Check sheet for the modelled part. Datum: model origin and axes. Units: mm. A direction names the side the tool comes from. Round coordinates to 2 decimals unless told otherwise and drop trailing zeros. Order: outer loops, then holes, each group sorted by start corner. A loop starts at its lowest first (then second) coordinate and runs counter-clockwise, first axis right, second up. Notation, with made-up numbers: (-12, 85.25) -> (35, 85.25) arc R33 ccw to (35, 118.25) -> close; hole circle Ø10 at (-31.5, 51.5). An arc over 180 degrees is marked (long way). Answer in a Markdown table with one row per item.
from build123d import *

# Parameters (mm, degrees)
F3_R     = 4.445
F4_DEPTH = 177.545717
F6_R     = 3.81
F7_DEPTH = 235.710434


with BuildPart() as f1:
    # F0 (on Top) → F1 (revolve)
    with BuildSketch(Plane.XY):
        Polygon((-12.572359, 12.572359), (-25.144717, 0), (-25.144717, -2.54), (0, -2.54), (0, 0), (0, 80.769434), (0, 83.309434), (-25.144717, 83.309434), (-25.144717, 80.769434), (-12.572359, 68.197076), (-12.572359, 55.497076), (-25.144717, 42.924717), (-25.144717, 40.384717), (-25.144717, 37.844717), (-12.572359, 25.272359), align=None)
    revolve(axis=Axis((0, 40.384717, 0), (0, -1, 0)))

    # F3 (on offset) → F4 (cut, through all)
    with BuildSketch(Plane.XY.offset(152.4)):
        with Locations((0.078337, 40.451534)):
            Circle(F3_R)
    extrude(amount=-F4_DEPTH, mode=Mode.SUBTRACT)

    # F6 (on offset) → F7 (cut, through all)
    with BuildSketch(Plane.XZ.offset(152.4)):
        with Locations((0.109616, -0.012402)):
            Circle(F6_R)
    extrude(amount=-F7_DEPTH, mode=Mode.SUBTRACT)


solid = f1.part
Item 1: Cross-section at C-C (y = 8). Record the boundary of the cut face in (x, z).
Result sheet:
| item | result |
|---|---|
| outline | circle Ø34.29 at (0, 0); hole circle Ø7.62 at (0.11, -0.01) |
Item 2: Cross-section at B-B (z = 18). State how many separate pieces and enclosed holes the cut face has, and give its area (3 significant figures).
Result sheet:
| item | result |
|---|---|
| separate pieces | 3 |
| enclosed holes | 1 |
| area | 941 mm^2 |
Item 3: Mould release check, pull along Y, two halves, no side actions. Record for faces 1 (the flat face through (0, 83.309, 5)), 2 (the conical face through (2.9, 54.71, 13.04)), 3 (the cylindrical face through (3.27, 82.02, -24.93)): pulls with the +Y half, pulls with the -Y half, needs draft (parallel to the pull), parting line crosses it, or undercut.
Result sheet:
| item | result |
|---|---|
| face 1 | pulls with the +Y half |
| face 2 | undercut |
| face 3 | needs draft |
Item 4: Set-up check for faces 4 (the conical face through (2.858, 25.883, 12.869)), 5 (the cylindrical face through (4.318, 41.787, 0.349)): record each of +Z, -Z, +X, -X, +Y, -Y from which the full face is reachable in a straight line by a thin tool's end or side.
Result sheet:
| item | result |
|---|---|
| face 4 | none |
| face 5 | +Z, -Z |
Item 5: Cross-section at A-A (x = 0). Record the boundary of the cut face in (y, z), and give its area (3 significant figures).
Result sheet:
| item | result |
|---|---|
| outline | (-2.54, -25.14) -> (0, -25.14) -> (12.57, -12.57) -> (25.27, -12.57) -> (36.01, -23.31) -> (36.01, -3.82) -> (-2.54, -3.82) -> close; (-2.54, 3.8) -> (36.01, 3.8) -> (36.01, 23.31) -> (25.27, 12.57) -> (12.57, 12.57) -> (0, 25.14) -> (-2.54, 25.14) -> close; (44.9, -23.17) -> (55.5, -12.57) -> (68.2, -12.57) -> (80.77, -25.14) -> (83.31, -25.14) -> (83.31, -3.82) -> (44.9, -3.82) -> close; (44.9, 3.8) -> (83.31, 3.8) -> (83.31, 25.14) -> (80.77, 25.14) -> (68.2, 12.57) -> (55.5, 12.57) -> (44.9, 23.17) -> close |
| area | 2,020 mm^2 |
Item 6: Scan lines: line 1 (Y direction, x = 17, z = -7); line 2 (Y direction, x = -2.5, z = -19.5); line 3 (Y direction, x = 16.5, z = 3.5). Record each from-to range of solid material in increasing order. Write a range as [from, to].
Result sheet:
| item | result |
|---|---|
| line 1 | y = [-2.54, 6.76], [31.08, 49.68], [74.01, 83.31] |
| line 2 | y = [-2.54, 5.49], [32.36, 36.83], [44.07, 48.41], [75.28, 83.31] |
| line 3 | y = [-2.54, 8.28], [29.57, 51.2], [72.49, 83.31] |
Item 7: Depth check by flat-ended pin: P1, Ø8, axis at y = 71, z = -17.5, coming from the -X side; P2, Ø8, axis at x = -1, y = 60.5, coming from the -Z side; P3, Ø6, axis at x = 0.11, z = -0.01, coming from the -Y side; P4, Ø10, axis at x = 5.5, y = 6.5, coming from the -Z side. Enter the tip coordinate at first touch or a pass-through.
Result sheet:
| item | result |
|---|---|
| P1 | stops at x = -10.82 |
| P2 | stops at z = -12.57 |
| P3 | passes through |
| P4 | stops at z = -23.11 |
